from build123d import *

# Parameters (mm, degrees)
SKETCH1_R           = 44.45
SKETCH1_R_2         = 31.75
BOSS_EXTRUDE1_DEPTH = 75
CIRPATTERN1_COUNT   = 6


with BuildPart() as part:
    # Sketch1 → Boss-Extrude1 (new body, symmetric)
    with BuildSketch(Plane.XY):
        Circle(SKETCH1_R)
        Circle(SKETCH1_R_2, mode=Mode.SUBTRACT)
    extrude(amount=BOSS_EXTRUDE1_DEPTH, both=True)

    # Sketch3 → M5x0.8 Tapped Hole1 (revolve, cut)
    with BuildSketch(Plane(origin=(0, 38.1, 75), x_dir=(0, -1, 0), z_dir=(1, 0, 0))):
        Polygon((0, 0), (0, 13.6618073), (2.1, 12.4), (2.1, 0), align=None)
    m5x0_8_tapped_hole1 = revolve(axis=Axis((0, 38.1, 81.35), (0, 0, -1)), mode=Mode.SUBTRACT)

    # CirPattern1: M5x0.8 Tapped Hole1 ×6 about axis
    cirpattern1_axis = Axis((0, 0, 0), (0, 0, 1))
    for i in range(1, CIRPATTERN1_COUNT):
        add(m5x0_8_tapped_hole1.rotate(cirpattern1_axis, i * 360 / CIRPATTERN1_COUNT), mode=Mode.SUBTRACT)

    # Mirror1: M5x0.8 Tapped Hole1 across plane
    add(m5x0_8_tapped_hole1.mirror(Plane.XY), mode=Mode.SUBTRACT)

    # Mirror1 copy 1 sketch → Mirror1 copy 1 (revolve, cut)
    with BuildSketch(Plane(origin=(-32.995567884, 19.05, -75), x_dir=(0.866025404, -0.5, 0), z_dir=(0.5, 0.866025404, 0))):
        Polygon((0, 0), (0, -13.6618073), (2.1, -12.4), (2.1, 0), align=None)
    revolve(axis=Axis((-32.995567884, 19.05, -81.35), (0, 0, -1)), mode=Mode.SUBTRACT)

    # Mirror1 copy 2 sketch → Mirror1 copy 2 (revolve, cut)
    with BuildSketch(Plane(origin=(-32.995567884, -19.05, -75), x_dir=(0.866025404, 0.5, 0), z_dir=(-0.5, 0.866025404, 0))):
        Polygon((0, 0), (0, -13.6618073), (2.1, -12.4), (2.1, 0), align=None)
    revolve(axis=Axis((-32.995567884, -19.05, -81.35), (0, 0, -1)), mode=Mode.SUBTRACT)

    # Mirror1 copy 3 sketch → Mirror1 copy 3 (revolve, cut)
    with BuildSketch(Plane(origin=(0, -38.1, -75), x_dir=(0, 1, 0), z_dir=(-1, 0, 0))):
        Polygon((0, 0), (0, -13.6618073), (2.1, -12.4), (2.1, 0), align=None)
    revolve(axis=Axis((0, -38.1, -81.35), (0, 0, -1)), mode=Mode.SUBTRACT)

    # Mirror1 copy 4 sketch → Mirror1 copy 4 (revolve, cut)
    with BuildSketch(Plane(origin=(32.995567884, -19.05, -75), x_dir=(-0.866025404, 0.5, 0), z_dir=(-0.5, -0.866025404, 0))):
        Polygon((0, 0), (0, -13.6618073), (2.1, -12.4), (2.1, 0), align=None)
    revolve(axis=Axis((32.995567884, -19.05, -81.35), (0, 0, -1)), mode=Mode.SUBTRACT)

    # Mirror1 copy 5 sketch → Mirror1 copy 5 (revolve, cut)
    with BuildSketch(Plane(origin=(32.995567884, 19.05, -75), x_dir=(-0.866025404, -0.5, 0), z_dir=(0.5, -0.866025404, 0))):
        Polygon((0, 0), (0, -13.6618073), (2.1, -12.4), (2.1, 0), align=None)
    revolve(axis=Axis((32.995567884, 19.05, -81.35), (0, 0, -1)), mode=Mode.SUBTRACT)


solid = part.part
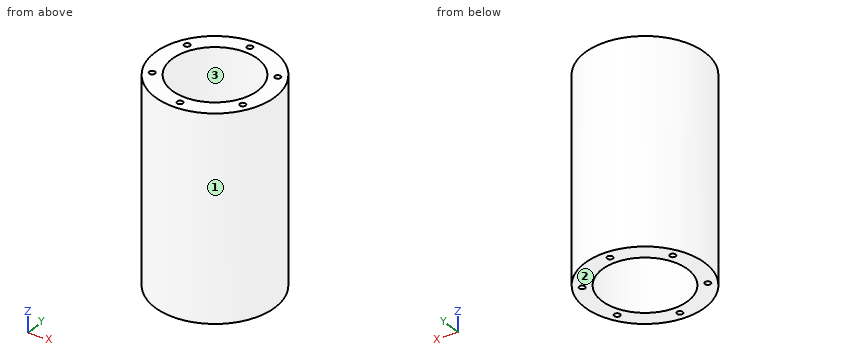
Read the model definition and answer for the solid it produces. Units are mm, in the model's axes. Face numbers are marked on the shaded views. Give positions to 0.01 mm unless a question says otherwise; leave off trailing zeros. Loops run counter-clockwise (first coordinate to the right, second up) from the corner with the lowest first, then second, coordinate; pieces in that order, holes last. Notation, with made-up numbers: (6.25, 68) - (44.25, 68) arc R36 ccw to (44.25, 105) - close; hole circle Ø8 at (85, -31.5). An arc over 180 degrees is marked (long way). Answer as CSV lines item,"result". Start each with the question number.
1) Determine the mould class of the marked faces 1, 2 and 3 for opening direction Y: released by +Y, released by -Y, zero draft, split by the parting line, or undercut.
2) Find section A-A (y = -24). Write down the section's boundary in (x, z), then the cut area to 3 significant figures.
3) Find section B-B (z = -47). Write down the section's boundary in (x, y), then the cut area to 3 significant figures.
4) Straight lines are drawn through the part: L1, parallel to X at y = -19, z = -72; L2, parallel to Y at x = 8.5, z = -45; L3, parallel to Y at x = -19, z = -46. For each, find the intervals that lie inside material, in ascending order. Write a range as from..to.
5) Find section C-C (x = 26.5). Write down the section's boundary in (y, z).
6) Each of these flat-tipped pins is pushed along its axis until it touches: pin 1 Ø5 at (x, z) = (-14, 52.5) entering from +Y; pin 2 Ø3.5 at (x, y) = (33, -19.05) entering from -Z; pin 3 Ø8 at (y, z) = (-8, 11) entering from +X. Where does it stop, or does it pass through?
Findings below:
1,face 1,"split by the parting line"
1,face 2,"zero draft"
1,face 3,"undercut"
2,outline,"(-37.41, -75) - (-20.79, -75) - (-20.79, 75) - (-37.41, 75) - close; (20.79, -75) - (37.41, -75) - (37.41, 75) - (20.79, 75) - close"
2,area,"4,990 mm^2"
3,outline,"circle Ø88.9 at (0, 0); hole circle Ø63.5 at (0, 0)"
3,area,"3,040 mm^2"
4,L1,"-40.18..-35.09, -30.9..-25.44, 25.44..30.9, 35.09..40.18"
4,L2,"-43.63..-30.59, 30.59..43.63"
4,L3,"-40.18..-25.44, 25.44..40.18"
5,outline,"(-35.69, -75) - (-17.49, -75) - (-17.49, 75) - (-35.69, 75) - close; (17.49, -75) - (35.69, -75) - (35.69, 75) - (17.49, 75) - close"
6,pin 1,"y = 42.94"
6,pin 2,"z = -62.39"
6,pin 3,"x = 44.27"
